Work out the finished part from the listing and answer in its coordinate system (mm). A direction names the side the tool comes from. Round coordinates to 2 decimals unless told otherwise and drop trailing zeros. Loops run counter-clockwise (first coordinate to the right, second up) from the corner with the lowest first, then second, coordinate; pieces in that order, holes last. Notation, with made-up numbers: (31, 87.25) - (87, 87.25) arc R21 ccw to (87, 107.25) - close; hole circle Ø3 at (75.5, -34.5). An arc over 180 degrees is marked (long way). Answer as CSV lines item,"result". Start each with the question number.
Q1. For faces 1 (the face through (0, -5.499, -51)), 2 (the face through (5, -3, -38.1)), 3 (the face through (-4.74, 2.79, -50.98)), determine the directions among +Z, -Z, +X, -X, +Y, -Y from which every point of the face is accessible in a straight line to the end or side of a thin tool.
Q2. Section B-B on x = 0 is taken. Write down the section's boundary in (y, z), then the cut area to 3 significant figures.
Q3. Section C-C on z = -45.5 is taken. Write down the section's boundary in (x, y) (3 decimals), then the cut area to 3 significant figures.
Q4. Section A-A on y = -3.75 is taken. Write down the section's boundary in (x, z).
Q5. The mould has two halves that part along Y. Classify faces 4 (the face through (-5, -3, -38.1)), 5 (the face through (4.785, 2.711, -50.978)), 6 (the face through (4.74, -2.79, -50.98)), 7 (the face through (-1.38, -6.2, 11.99)): +Y half, -Y half, draft (parallel to the pull), parting line (faces both ways), or undercut.
Q6. Each of these flat-tipped pins is pushed along its axis until it touches: pin 1 Ø1 at (x, z) = (4.5, -40) entering from -Y; pin 2 Ø1 at (x, y) = (5.5, -4) entering from -Z; pin 3 Ø3 at (x, z) = (-1.5, -55) entering from +Y. Where does it stop, or does it pass through?
Q7. Section D-D on z = 24 is taken. Write down the section's boundary in (x, y).
Q8. Straight lines are drawn through the part: L1, parallel to Y at x = 0.5, z = -1; L2, parallel to Y at x = -5.5, z = 6; L3, parallel to Z at x = -5, y = 2.5. For each, find the intervals that lie inside material, in ascending order. Write a range as [from, to].
```python
from build123d import *

# Parameters (mm, degrees)
BOSS_EXTRUDE1_DEPTH      = 63.5
BOSS_EXTRUDE1_DEPTH_BACK = 63.5
SKETCH1_R                = 6.35
CUT_EXTRUDE1_DEPTH       = 25.4


with BuildPart() as part:
    # Sketch1 → Boss-Extrude1 (new, two sides: drawn at the far end of the back side and taken through both)
    with BuildSketch(Plane.XY.offset(-BOSS_EXTRUDE1_DEPTH_BACK)):
        Circle(SKETCH1_R)
    extrude(amount=BOSS_EXTRUDE1_DEPTH + BOSS_EXTRUDE1_DEPTH_BACK)

    # Sketch2 → Cut-Extrude1 (cut)
    with BuildSketch(Plane(origin=(0, 0, -63.5), x_dir=(-1, 0, 0), z_dir=(0, 0, -1))):
        with BuildLine():
            ThreePointArc((6.35, 0), (5.499261314, 3.175), (3.175, 5.499261314))
            Line((3.175, 5.499261314), (6.35, 0))
        make_face()
        with BuildLine():
            Line((-3.175, 5.499261314), (3.175, 5.499261314))
            ThreePointArc((3.175, 5.499261314), (0, 6.35), (-3.175, 5.499261314))
        make_face()
        with BuildLine():
            Line((-6.35, 0), (-3.175, 5.499261314))
            ThreePointArc((-3.175, 5.499261314), (-5.499261314, 3.175), (-6.35, 0))
        make_face()
        with BuildLine():
            ThreePointArc((3.175, -5.499261314), (5.499261314, -3.175), (6.35, 0))
            Line((6.35, 0), (3.175, -5.499261314))
        make_face()
        with BuildLine():
            Line((-3.175, -5.499261314), (-6.35, 0))
            ThreePointArc((-6.35, 0), (-5.499261314, -3.175), (-3.175, -5.499261314))
        make_face()
        with BuildLine():
            ThreePointArc((-3.175, -5.499261314), (0, -6.35), (3.175, -5.499261314))
            Line((3.175, -5.499261314), (-3.175, -5.499261314))
        make_face()
    extrude(amount=-CUT_EXTRUDE1_DEPTH, mode=Mode.SUBTRACT)


solid = part.part
```
Findings:
1,face 1,"-Z, +X, -X, -Y"
1,face 2,"-Z, +X, -Y"
1,face 3,"-Z, -X, +Y"
2,outline,"(-6.35, -38.1) - (-5.5, -38.1) - (-5.5, -63.5) - (5.5, -63.5) - (5.5, -38.1) - (6.35, -38.1) - (6.35, 63.5) - (-6.35, 63.5) - close"
2,area,"1,570 mm^2"
3,outline,"(-6.35, 0) - (-3.175, -5.499) - (3.175, -5.499) - (6.35, 0) - (3.175, 5.499) - (-3.175, 5.499) - close"
3,area,"105 mm^2"
4,outline,"(-5.12, -38.1) - (-4.18, -38.1) - (-4.18, -63.5) - (4.18, -63.5) - (4.18, -38.1) - (5.12, -38.1) - (5.12, 63.5) - (-5.12, 63.5) - close"
5,face 4,"draft"
5,face 5,"+Y half"
5,face 6,"-Y half"
5,face 7,"parting line"
6,pin 1,"stops at y = -4.07"
6,pin 2,"stops at z = -38.1"
6,pin 3,"stops at y = 5.5"
7,outline,"circle Ø12.7 at (0, 0)"
8,L1,"y = [-6.33, 6.33]"
8,L2,"y = [-3.17, 3.17]"
8,L3,"z = [-38.1, 63.5]"
